```python
from build123d import *

# Parameters (mm, degrees)
F1_W     = 36
F1_H     = 8
F3_DEPTH = 2
F0_R     = 1.15
F4_DEPTH = 2.001
F5_DEPTH = 1.4
F6_R     = 3.99999


# Not quite as in the source:
# - a fillet or chamfer is up to 0.001 mm smaller than in the source, because OpenCascade refuses the exact size


with BuildPart() as f3:
    # F1 (on Top) → F3 (new body)
    with BuildSketch(Plane.XY):
        Rectangle(F1_W, F1_H)
    extrude(amount=F3_DEPTH)

    # F0 (on Top) → F4 (cut, through all)
    with BuildSketch(Plane.XY):
        with Locations((-13, 0)):
            Circle(F0_R)
        with Locations((13, 0)):
            Circle(F0_R)
    extrude(amount=F4_DEPTH, mode=Mode.SUBTRACT)

    # F2 (on Top) → F5 (cut)
    with BuildSketch(Plane.XY):
        Polygon((-11.8943742345, -1.915), (-10.788748469, 0), (-11.8943742345, 1.915), (-13, 1.915), (-14.1056257655, 1.915), (-15.211251531, 0), (-14.1056257655, -1.915), (-13, -1.915), align=None)
        Polygon((14.1056257655, -1.915), (15.211251531, 0), (14.1056257655, 1.915), (13, 1.915), (11.8943742345, 1.915), (10.788748469, 0), (11.8943742345, -1.915), (13, -1.915), align=None)
    extrude(amount=F5_DEPTH, mode=Mode.SUBTRACT)

    # F6 (radius 4 in the source; OpenCascade refuses exactly that, so slightly less here)
    f6_edges = [f3.edges().sort_by_distance(p)[0] for p in [
        (-18, 4, 1),
        (-18, -4, 1),
        (18, -4, 1),
        (18, 4, 1),
    ]]
    fillet(f6_edges, radius=F6_R)


solid = f3.part
```
Model file for the job. Use its own axes, mm. A direction names the side the tool comes from. Round coordinates to 2 decimals unless told otherwise and drop trailing zeros. Write each loop counter-clockwise with the first axis right and the second up, starting at its lowest first coordinate (ties: lowest second). Pieces come first, ordered by that corner, then holes. Notation, with made-up numbers: (67, -18.5) - (76, -18.5) arc R17 cw to (76, 4.5) - close; hole circle Ø10 at (59.25, 20). An arc over 180 degrees is marked (long way). One line per item, written item: value.
(1) Two-plate mould, pull along X, no slides. Class faces 1 (the flat face through (14, 1, 1.4)), 2 (the cylindrical face through (16.797, -2.859, 1.014)), 3 (the flat face through (0, 0, 2)): pulls with the +X half, pulls with the -X half, needs draft (parallel to the pull), parting line crosses it, or undercut.
Values follow:
face 1: undercut
face 2: pulls with the +X half
face 3: needs draft
(2) Wall check: probe 1 along X at (y, z) = (0, 1.7); probe 2 along Y at (x, z) = (13, 1.5); probe 3 along Y at (x, z) = (13, 0.2) (3 decimals). Give the ranges that are in metal, low to high.
Values follow:
probe 1: x = -18 to -14.15, -11.85 to 11.85, 14.15 to 18
probe 2: y = -4 to -1.15, 1.15 to 4
probe 3: y = -4 to -1.915, 1.915 to 4
(3) Cut at A-A, the plane x = -13. Give the cut face in (y, z) (3 decimals).
Values follow:
outline: (-4, 0) - (-1.915, 0) - (-1.915, 1.4) - (-1.15, 1.4) - (-1.15, 2) - (-4, 2) - close; (1.15, 1.4) - (1.915, 1.4) - (1.915, 0) - (4, 0) - (4, 2) - (1.15, 2) - close
(4) Cut at D-D, the plane y = 3.25. Give the cut face in (x, z), plus the area to 3 significant figures.
Values follow:
outline: (-16.33, 0) - (16.33, 0) - (16.33, 2) - (-16.33, 2) - close
area: 65.3 mm²
(5) 3-axis set-ups, long thin cutter, end or side, ignore diameter. For faces 4 (the cylindrical face through (14.097, 0.345, 1.696)), 5 (the flat face through (-11.33, 0.94, 0.69)): which of +Z, -Z, +X, -X, +Y, -Y reach the whole face in a straight line?
Values follow:
face 4: +Z, -Z
face 5: -Z
(6) Cut at B-B, the plane z = 1.7. Give the number of separate pieces and of enclosed holes in the cut face, plus the area to 3 significant figures.
Values follow:
separate pieces: 1
enclosed holes: 2
area: 266 mm²
(7) Drop a flat-ended pin along its axis: P1, Ø2.5, axis at x = -13, y = 0, coming from the +Z side. Give the stop position or say it passes through.
Values follow:
P1: stops at z = 2
(8) Cut at C-C, the plane y = -0.5. Give the cut face in (x, z).
Values follow:
outline: (-17.97, 0) - (-14.92, 0) - (-14.92, 1.4) - (-14.04, 1.4) - (-14.04, 2) - (-17.97, 2) - close; (-11.96, 1.4) - (-11.08, 1.4) - (-11.08, 0) - (11.08, 0) - (11.08, 1.4) - (11.96, 1.4) - (11.96, 2) - (-11.96, 2) - close; (14.04, 1.4) - (14.92, 1.4) - (14.92, 0) - (17.97, 0) - (17.97, 2) - (14.04, 2) - close
